Read the model definition and answer for the solid it produces. Units are mm, in the model's axes. A direction names the side the tool comes from. Give positions to 0.01 mm unless a question says otherwise; leave off trailing zeros. Write each loop counter-clockwise with the first axis right and the second up, starting at its lowest first coordinate (ties: lowest second). Pieces come first, ordered by that corner, then holes. Notation, with made-up numbers: M 54,75.25 L 80,75.25 A35 cw 80,110.25 Z; hole C -24.75,31.5 d9. An arc over 180 degrees is marked long. Put each result on its own line as item: value.
from build123d import *

# Parameters (mm, degrees)
ESQUISSE1_R             = 6.8
BOSS_EXTRU_1_DEPTH      = 15
COQUE1_T                = -1
ESQUISSE2_R             = 3.55
ENL_V_MAT_EXTRU_1_DEPTH = 15
CHANFREIN1_SIZE         = 3
BOSS_EXTRU_2_DEPTH      = 5
BOSS_EXTRU_3_DEPTH      = 1
BOSS_EXTRU_4_START      = -3
ESQUISSE5_R             = 7.8
ESQUISSE5_R_2           = 6.8
BOSS_EXTRU_4_DEPTH      = 1


with BuildPart() as part:
    # Esquisse1 → Boss.-Extru.1 (new body)
    with BuildSketch(Plane.XY):
        Circle(ESQUISSE1_R)
    extrude(amount=BOSS_EXTRU_1_DEPTH)

    # Coque1
    coque1_openings = [part.faces().sort_by_distance(p)[0] for p in [
        (0, 0, 15),
    ]]
    offset(amount=COQUE1_T, openings=coque1_openings, kind=Kind.INTERSECTION)

    # Esquisse2 → Enlèv. mat.-Extru.1 (cut)
    with BuildSketch(Plane(origin=(0, 0, 0), x_dir=(-1, 0, 0), z_dir=(0, 0, -1))):
        Circle(ESQUISSE2_R)
    extrude(amount=-ENL_V_MAT_EXTRU_1_DEPTH, mode=Mode.SUBTRACT)

    # Chanfrein1
    # the kernel refuses this chamfer: 3 mm, written as the material it adds along each edge
    with BuildSketch(Plane(origin=(0, 0, 1), x_dir=(1, 0, 0), z_dir=(0, 1, 0))) as chanfrein1_piece_1_section:
        Polygon((5.8, -CHANFREIN1_SIZE), (5.8 - CHANFREIN1_SIZE, 0), (5.8, 0), align=None)
    chanfrein1_piece_1 = revolve(axis=Axis((0, 0, 1), (0, 0, -1)), mode=Mode.PRIVATE)
    chanfrein1_piece_1 = chanfrein1_piece_1 - Plane(origin=(0, 0, 2.8805317), x_dir=(-1, 0, 0), z_dir=(0, 0, -1)) * Cylinder(3.55, 24, mode=Mode.PRIVATE)
    add(chanfrein1_piece_1)

    # Esquisse3 → Boss.-Extru.2 (add)
    with BuildSketch(Plane(origin=(0, 0, 0), x_dir=(-1, 0, 0), z_dir=(0, 0, -1))):
        with BuildLine():
            Line((-6.726068688, 1), (-10, 1))
            Line((-10, 1), (-10, -1))
            Line((-10, -1), (-6.726068688, -1))
            ThreePointArc((-6.726068688, -1), (-6.8, 0), (-6.726068688, 1))
        make_face()
        with BuildLine():
            Line((10, -1), (6.726068688, -1))
            ThreePointArc((6.726068688, -1), (6.8, 0), (6.726068688, 1))
            Line((6.726068688, 1), (10, 1))
            Line((10, 1), (10, -1))
        make_face()
    extrude(amount=-BOSS_EXTRU_2_DEPTH)

    # Esquisse4 → Boss.-Extru.3 (add)
    with BuildSketch(Plane.XY.offset(5)):
        with BuildLine():
            Line((10, 2), (10, -2))
            Line((10, -2), (6.499230724, -2))
            Line((6.499230724, -2), (5.444263036, -2))
            ThreePointArc((5.444263036, -2), (5.8, 0), (5.444263036, 2))
            Line((5.444263036, 2), (6.499230724, 2))
            Line((6.499230724, 2), (10, 2))
        make_face()
    extrude(amount=BOSS_EXTRU_3_DEPTH)

    # Esquisse5 → Boss.-Extru.4 (add)
    with BuildSketch(Plane.XY.offset(15).offset(BOSS_EXTRU_4_START)):
        Circle(ESQUISSE5_R)
        with Locations(Location((0, 0, 0), (0, 0, 171.543480665))):
            Circle(ESQUISSE5_R_2, mode=Mode.SUBTRACT)
    extrude(amount=BOSS_EXTRU_4_DEPTH)


solid = part.part
(1) Section A-A on x = 0 is taken. Determine the outline of the cut face in (y, z).
Result:
outline: M -7.8,12 L -6.8,12 L -6.8,0 L -3.55,0 L -3.55,1.75 L -5.8,4 L -5.8,15 L -6.8,15 L -6.8,13 L -7.8,13 Z; M 3.55,0 L 6.8,0 L 6.8,12 L 7.8,12 L 7.8,13 L 6.8,13 L 6.8,15 L 5.8,15 L 5.8,4 L 3.55,1.75 Z
(2) For a pull along Z with two mould halves and no side action, classify faces 5 (the face through (-8, 0, 5)), 6 (the face through (-8, 1, 2)), 7 (the face through (1, 7, 12)), 8 (the face through (8.3, -1.5, 5)) as +Z half, -Z half, draft (parallel to the pull), parting line (faces both ways), or undercut.
Result:
face 5: undercut
face 6: draft
face 7: undercut
face 8: -Z half
(3) Given pin 1 Ø3.5 at (x, z) = (-9, 1.5) entering from -Y; pin 2 Ø1 at (x, z) = (7.5, 3) entering from +Y; pin 3 Ø0.8 at (x, y) = (8, 1.5) entering from -Z, each flat-ended and moving along its own axis, determine where each tip first touches the part or whether it passes through.
Result:
pin 1: stops at y = -1
pin 2: stops at y = 1
pin 3: stops at z = 5
(4) Which of the six approach directions +Z, -Z, +X, -X, +Y, -Y give full straight-line access (tool end or side, diameter ignored) to faces 1 (the face through (-8, -1, 2)), 2 (the face through (8.3, -2, 5.5)), 3 (the face through (-5.794, 0.255, 9.423)), 4 (the face through (8.3, 1.5, 5))?
Result:
face 1: -Z, -X, -Y
face 2: -Z, +X, -Y
face 3: +Z
face 4: -Z, +X, +Y
(5) Section D-D on x = 7.5 is taken. Determine the outline of the cut face in (y, z).
Result:
outline: M -2.14,12 L 2.14,12 L 2.14,13 L -2.14,13 Z; M -2,5 L -1,5 L -1,0 L 1,0 L 1,5 L 2,5 L 2,6 L -2,6 Z
(6) Section C-C on z = 4.5 is taken. Determine the outline of the cut face in (x, y).
Result:
outline: M -10,-1 L -6.73,-1 A6.8 ccw 6.73,-1 L 10,-1 L 10,1 L 6.73,1 A6.8 ccw -6.73,1 L -10,1 Z; hole C 0,0 d11.6
(7) Section B-B on y = 0 is taken. Determine the outline of the cut face in (x, z).
Result:
outline: M -10,0 L -3.55,0 L -3.55,1.75 L -5.8,4 L -5.8,15 L -6.8,15 L -6.8,13 L -7.8,13 L -7.8,12 L -6.8,12 L -6.8,5 L -10,5 Z; M 3.55,0 L 10,0 L 10,6 L 6.8,6 L 6.8,12 L 7.8,12 L 7.8,13 L 6.8,13 L 6.8,15 L 5.8,15 L 5.8,4 L 3.55,1.75 Z
(8) Straight lines are drawn through the part: line 1 along Y through (x, z) = (0, 0.85); line 2 along X through (y, z) = (0, 11). For each, find the intervals that lie inside material, in ascending order. Write a range as from..to.
Result:
line 1: y = -6.8..-3.55, 3.55..6.8
line 2: x = -6.8..-5.8, 5.8..6.8
